from build123d import *


# Not quite as in the source:
# - ends of sketch curves that miss each other by under 0.0002 mm in the source are joined


with BuildPart() as f1:
    # F0 (on Front) → F1 (revolve)
    with BuildSketch(Plane.XZ):
        with BuildLine():
            Line((0, 4.9999998882), (0, 0))
            Line((0, 0), (23.0616367864, 0))
            ThreePointArc((23.0616367864, 0), (28.3032507173, 1.95636836), (30.9812327357, 6.8686291501))
            Line((30.9812327357, 6.8686291501), (39.6738796125, 67.7171572875))
            ThreePointArc((39.6738796125, 67.7171572875), (39.2048885352, 69.3104034827), (37.6939806252, 70))
            Line((37.6939806252, 70), (36.6838267834, 70))
            ThreePointArc((36.6838267834, 70), (35.3734233007, 69.51090791), (34.7039277961, 68.2828427125))
            Line((34.7039277961, 68.2828427125), (26.0314839961, 7.5757361129))
            ThreePointArc((26.0314839961, 7.5757361129), (25.0272421924, 5.7336379253), (23.0616367864, 4.9999997224))
            Line((23.0616367864, 4.9999997224), (0, 4.9999998882))
        make_face()
    revolve(axis=Axis((0, 0, 2.4999999441), (0, 0, -1)))


solid = f1.part
Could you check a few things on this model? Use its own coordinates, in mm. Round coordinates to 2 decimals unless told otherwise and drop trailing zeros. Order: outer loops, then holes, each group sorted by start corner. A loop starts at its lowest first (then second) coordinate and runs counter-clockwise, first axis right, second up.
Q1. Thinking about a two-plate mould opening in Y: for faces 1 (the face through (32.833, -10.34, 30.958)), 2 (the face through (0, 0, 0)), 3 (the face through (-6.361, 28.646, 30.759)), which applies, released by +Y, released by -Y, zero draft, split by the parting line, or undercut?
Geometry says:
face 1: split by the parting line
face 2: zero draft
face 3: undercut
Q2. Imagine slicing it at B-B, the plane z = 51.5. List the corners of the cut face in (x, y) for me, then the cut area to 3 significant figures.
Geometry says:
outline: circle Ø74.71 at (0, 0); hole circle Ø64.61 at (0, 0)
area: 1,110 mm2
Q3. Please list where these lines run through material, in increasing order: probe 1 along Y at (x, z) = (-21, 29.5); probe 2 along X at (y, z) = (21, 32.5); probe 3 along X at (y, z) = (15, 61.5).
Geometry says:
probe 1: y = -27.01 to -20.24, 20.24 to 27.01
probe 2: x = -27.55 to -20.85, 20.85 to 27.55
probe 3: x = -35.77 to -30.22, 30.22 to 35.77
Q4. I'm going to push flat-ended pins straight in: P1, Ø12, axis at y = -29.5, z = 49.5, coming from the +X side; P2, Ø4, axis at x = -29, z = 7.5, coming from the -Y side; P3, Ø8, axis at y = 9.5, z = 59, coming from the +X side. Where does each tip first touch, or does it pass through?
Geometry says:
P1: stops at x = 28.79
P2: stops at y = -15.42
P3: stops at x = 38.26
Q5. Imagine slicing it at A-A, the plane z = 44. List the corners of the cut face in (x, y) for me, then the cut area to 3 significant figures.
Geometry says:
outline: circle Ø72.57 at (0, 0); hole circle Ø62.47 at (0, 0)
area: 1,070 mm2
